The listing builds one solid part. Answer for the finished solid, in the listing's coordinates (mm). Face numbers are marked on the shaded views. A direction names the side the tool comes from. Give positions to 0.01 mm unless a question says otherwise; leave off trailing zeros. Order: outer loops, then holes, each group sorted by start corner. A loop starts at its lowest first (then second) coordinate and runs counter-clockwise, first axis right, second up. Notation, with made-up numbers: (-31, -36) - (11, -36) arc R15 ccw to (11, -28) - close; hole circle Ø7 at (12.25, 44). An arc over 180 degrees is marked (long way). Answer in a Markdown table with one row per item.
from build123d import *

# Parameters (mm, degrees)
CROQUIS1_R              = 20
CROQUIS1_R_2            = 10
SALIENTE_EXTRUIR1_DEPTH = 2.75
CORTAR_EXTRUIR1_START   = -2.5
CROQUIS2_R              = 20
CROQUIS2_R_2            = 19
CROQUIS2_R_3            = 18
CROQUIS2_R_4            = 17
CROQUIS2_R_5            = 16
CROQUIS2_R_6            = 15
CROQUIS2_R_7            = 14
CROQUIS2_R_8            = 13
CROQUIS2_R_9            = 12
CROQUIS2_R_10           = 11
CORTAR_EXTRUIR1_DEPTH   = 2.5
SALIENTE_EXTRUIR2_DEPTH = 2.75


with BuildPart() as part:
    # Croquis1 → Saliente-Extruir1 (new body)
    with BuildSketch(Plane.XY):
        Circle(CROQUIS1_R)
        Circle(CROQUIS1_R_2, mode=Mode.SUBTRACT)
    extrude(amount=SALIENTE_EXTRUIR1_DEPTH)

    # Croquis2 → Cortar-Extruir1 (cut)
    # profile 1 of 5: a face of its own
    with BuildSketch(Plane.XY.offset(2.75).offset(CORTAR_EXTRUIR1_START)):
        Circle(CROQUIS2_R)
        Circle(CROQUIS2_R_2, mode=Mode.SUBTRACT)
    # profile 2 of 5: a face of its own
    with BuildSketch(Plane.XY.offset(2.75).offset(CORTAR_EXTRUIR1_START)):
        Circle(CROQUIS2_R_3)
        Circle(CROQUIS2_R_4, mode=Mode.SUBTRACT)
    # profile 3 of 5: a face of its own
    with BuildSketch(Plane.XY.offset(2.75).offset(CORTAR_EXTRUIR1_START)):
        Circle(CROQUIS2_R_5)
        Circle(CROQUIS2_R_6, mode=Mode.SUBTRACT)
    # profile 4 of 5: a face of its own
    with BuildSketch(Plane.XY.offset(2.75).offset(CORTAR_EXTRUIR1_START)):
        Circle(CROQUIS2_R_7)
        Circle(CROQUIS2_R_8, mode=Mode.SUBTRACT)
    # profile 5 of 5: a face of its own
    with BuildSketch(Plane.XY.offset(2.75).offset(CORTAR_EXTRUIR1_START)):
        Circle(CROQUIS2_R_9)
        Circle(CROQUIS2_R_10, mode=Mode.SUBTRACT)
    extrude(amount=CORTAR_EXTRUIR1_DEPTH, mode=Mode.SUBTRACT)

    # Croquis3 → Saliente-Extruir2 (add)
    with BuildSketch(Plane.XY.offset(2.75)):
        Polygon((-2.222048604, 9.75), (0, 9.75), (2.222048604, 9.75), (2.222048604, 20.446693488), (-2.222048604, 20.446693488), align=None)
    extrude(amount=-SALIENTE_EXTRUIR2_DEPTH)


solid = part.part
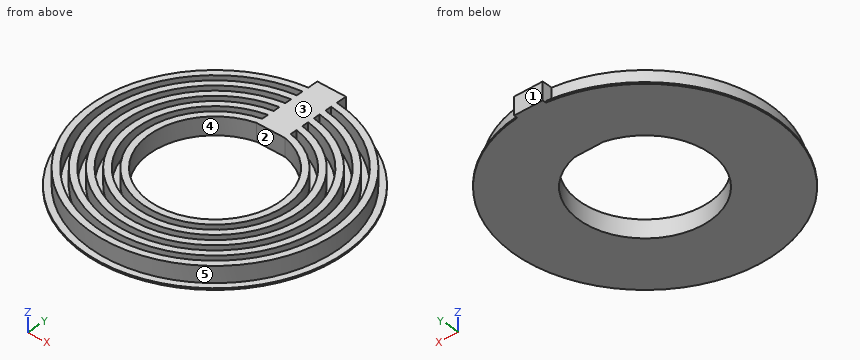
Item 1: Which of the six approach directions +Z, -Z, +X, -X, +Y, -Y give full straight-line access (tool end or side, diameter ignored) to the marked faces 1 and 2?
Answer block:
| item | result |
|---|---|
| face 1 | +Z, -Z, +X, -X, +Y |
| face 2 | +Z, -Z |
Item 2: Find section D-D on x = -15.5. Write down the section's boundary in (y, z), then the cut area to 3 significant figures.
Answer block:
| item | result |
|---|---|
| outline | (-12.64, 0) - (12.64, 0) - (12.64, 0.25) - (10.99, 0.25) - (10.99, 2.75) - (9.15, 2.75) - (9.15, 0.25) - (6.98, 0.25) - (6.98, 2.75) - (3.97, 2.75) - (3.97, 0.25) - (-3.97, 0.25) - (-3.97, 2.75) - (-6.98, 2.75) - (-6.98, 0.25) - (-9.15, 0.25) - (-9.15, 2.75) - (-10.99, 2.75) - (-10.99, 0.25) - (-12.64, 0.25) - close |
| area | 30.6 mm² |
Item 3: Determine the mould class of the marked faces 3, 4 and 5 for opening direction X: pulls with the +X half, pulls with the -X half, needs draft (parallel to the pull), parting line crosses it, or undercut.
Answer block:
| item | result |
|---|---|
| face 3 | needs draft |
| face 4 | undercut |
| face 5 | parting line crosses it |
Item 4: Find section A-A on x = 0. Write down the section's boundary in (y, z), then the cut area to 3 significant figures.
Answer block:
| item | result |
|---|---|
| outline | (-20, 0) - (-10, 0) - (-10, 2.75) - (-11, 2.75) - (-11, 0.25) - (-12, 0.25) - (-12, 2.75) - (-13, 2.75) - (-13, 0.25) - (-14, 0.25) - (-14, 2.75) - (-15, 2.75) - (-15, 0.25) - (-16, 0.25) - (-16, 2.75) - (-17, 2.75) - (-17, 0.25) - (-18, 0.25) - (-18, 2.75) - (-19, 2.75) - (-19, 0.25) - (-20, 0.25) - close; (9.75, 0) - (20.45, 0) - (20.45, 2.75) - (9.75, 2.75) - close |
| area | 44.4 mm² |
Item 5: Find section B-B on z = 1.4. Write down the section's boundary in (x, y).
Answer block:
| item | result |
|---|---|
| outline | (-2.22, 18.87) arc R19 ccw (long way) to (2.22, 18.87) - (2.22, 20.45) - (-2.22, 20.45) - close; hole (-2.22, 9.75) arc R10 ccw (long way) to (2.22, 9.75) - close; hole (-2.22, 10.77) - (-2.22, 11.79) arc R12 ccw (long way) to (2.22, 11.79) - (2.22, 10.77) arc R11 cw (long way) to start; hole (-2.22, 12.81) - (-2.22, 13.82) arc R14 ccw (long way) to (2.22, 13.82) - (2.22, 12.81) arc R13 cw (long way) to start; hole (-2.22, 14.83) - (-2.22, 15.84) arc R16 ccw (long way) to (2.22, 15.84) - (2.22, 14.83) arc R15 cw (long way) to start; hole (-2.22, 16.85) - (-2.22, 17.86) arc R18 ccw (long way) to (2.22, 17.86) - (2.22, 16.85) arc R17 cw (long way) to start |
Item 6: Each of these flat-tipped pins is pushed along its axis until it touches: P1, Ø1.1, axis at y = 17.5, z = 2, coming from the +X side; P2, Ø1.1, axis at y = 13.5, z = 1, coming from the -X side; P3, Ø0.5, axis at y = 15, z = 1, coming from the -X side. Where does it stop, or does it pass through?
Answer block:
| item | result |
|---|---|
| P1 | x = 8.58 |
| P2 | x = -13.9 |
| P3 | x = -11.98 |
Item 7: Consider line 1 (Y direction, x = 0, z = 1.5); line 2 (Z direction, x = -14.5, y = 4); line 3 (Y direction, x = 2, z = 0.8). Determine where each line is inside the solid, lowest interval first.
Answer block:
| item | result |
|---|---|
| line 1 | -19 to -18, -17 to -16, -15 to -14, -13 to -12, -11 to -10, 9.75 to 20.45 |
| line 2 | 0 to 0.25 |
| line 3 | -18.89 to -17.89, -16.88 to -15.87, -14.87 to -13.86, -12.85 to -11.83, -10.82 to -9.8, 9.75 to 20.45 |
